from build123d import *

# Parameters (mm, degrees)
SALIENTE_EXTRUIR1_DEPTH = 18
SALIENTE_EXTRUIR6_START = -36
SALIENTE_EXTRUIR6_DEPTH = 66
CORTAR_EXTRUIR1_START   = 48
CORTAR_EXTRUIR1_DEPTH   = 46
CORTAR_EXTRUIR2_START   = 18
CROQUIS4_R              = 25
CORTAR_EXTRUIR2_DEPTH   = 340.524582953
CROQUIS5_W              = 115
CROQUIS5_H              = 90
SALIENTE_EXTRUIR7_DEPTH = 34.5
CORTAR_EXTRUIR3_START   = 72
CROQUIS7_R              = 20
CORTAR_EXTRUIR3_DEPTH   = 398.972479579


with BuildPart() as part:
    # Croquis1 → Saliente-Extruir1 (new, symmetric)
    with BuildSketch(Plane(origin=(0, 0, 0), x_dir=(1, 0, 0), z_dir=(0, 1, 0))):
        with BuildLine():
            Line((-194.323843522, -100.327234865), (201.676156478, -100.327234865))
            ThreePointArc((201.676156478, -100.327234865), (301.676156478, -0.327234865), (201.676156478, 99.672765135))
            Line((201.676156478, 99.672765135), (-194.323843522, 99.672765135))
            ThreePointArc((-194.323843522, 99.672765135), (-294.323843522, -0.327234865), (-194.323843522, -100.327234865))
        make_face()
    extrude(amount=SALIENTE_EXTRUIR1_DEPTH, both=True)

    # Croquis2 → Saliente-Extruir6 (add)
    with BuildSketch(Plane(origin=(0, 18, 0), x_dir=(1, 0, 0), z_dir=(0, 1, 0)).offset(SALIENTE_EXTRUIR6_START)):
        with BuildLine():
            Line((-194.323843522, -75.327234865), (201.676156478, -75.327234865))
            ThreePointArc((201.676156478, -75.327234865), (276.676156478, -0.327234865), (201.676156478, 74.672765135))
            Line((201.676156478, 74.672765135), (-194.323843522, 74.672765135))
            ThreePointArc((-194.323843522, 74.672765135), (-269.323843522, -0.327234865), (-194.323843522, -75.327234865))
        make_face()
    extrude(amount=SALIENTE_EXTRUIR6_DEPTH)

    # Croquis3 → Cortar-Extruir1 (cut)
    with BuildSketch(Plane(origin=(0, 0, 0), x_dir=(1, 0, 0), z_dir=(0, 1, 0)).offset(CORTAR_EXTRUIR1_START)):
        with BuildLine():
            Line((-194.323843522, -50.327234865), (201.676156478, -50.327234865))
            ThreePointArc((201.676156478, -50.327234865), (251.676156478, -0.327234865), (201.676156478, 49.672765135))
            Line((201.676156478, 49.672765135), (-194.323843522, 49.672765135))
            ThreePointArc((-194.323843522, 49.672765135), (-244.323843522, -0.327234865), (-194.323843522, -50.327234865))
        make_face()
    extrude(amount=-CORTAR_EXTRUIR1_DEPTH, mode=Mode.SUBTRACT)

    # Croquis4 → Cortar-Extruir2 (cut, through all)
    with BuildSketch(Plane(origin=(0, 0, 0), x_dir=(1, 0, 0), z_dir=(0, 1, 0)).offset(CORTAR_EXTRUIR2_START)):
        with Locations(Location((-194.323843522, -0.327234865, 0), (0, 0, 90))):
            Circle(CROQUIS4_R)
        with Locations(Location((201.676156478, -0.327234865, 0), (0, 0, 90))):
            Circle(CROQUIS4_R)
    extrude(amount=-CORTAR_EXTRUIR2_DEPTH, mode=Mode.SUBTRACT)

    # Croquis5 → Saliente-Extruir7 (add, symmetric)
    with BuildSketch(Plane.XY):
        with Locations((14.961556785, 27)):
            Rectangle(CROQUIS5_W, CROQUIS5_H)
    extrude(amount=SALIENTE_EXTRUIR7_DEPTH, both=True)

    # Croquis7 → Cortar-Extruir3 (cut, through all)
    with BuildSketch(Plane(origin=(0, 0, 0), x_dir=(1, 0, 0), z_dir=(0, 1, 0)).offset(CORTAR_EXTRUIR3_START)):
        with Locations(Location((12.367095305, 2.963956449, 0), (0, 0, 270))):
            Circle(CROQUIS7_R)
    extrude(amount=-CORTAR_EXTRUIR3_DEPTH, mode=Mode.SUBTRACT)


solid = part.part
For this review, take the finished solid that the model builds, in its own axes (mm). A direction names the side the tool comes from. Give positions to 0.01 mm unless a question says otherwise; leave off trailing zeros. Order: outer loops, then holes, each group sorted by start corner. A loop starts at its lowest first (then second) coordinate and runs counter-clockwise, first axis right, second up. Notation, with made-up numbers: (85, -33.75) - (141, -33.75) arc R28 cw to (141, 3.25) - close; hole circle Ø3 at (40.25, -31.75). An arc over 180 degrees is marked (long way). Answer as a JSON object with one key per item and string values. Group by question number.
Item 1: Machinability: for faces 1 (the flat face through (1, 33, 75.327)), 2 (the flat face through (1, 0, 100.327)), 3 (the flat face through (14, 37, -34.5)), which of the approach directions +Z, -Z, +X, -X, +Y, -Y give a long, thin tool a straight path to every point of the face, cutting with its end or side? Answer none if there is none.
Item 2: Wall thickness on line 1 along Z through (x, y) = (39, 30); line 2 along Z through (x, y) = (143.5, 19); line 3 along X through (y, z) = (19, -20.5): over which ranges is each line inside the solid? List them lowest first.
Item 3: Take a section at D-D on x = -203.5. Give the boundary of the cut face in (y, z).
Item 4: Take a section at B-B on x = -37. Give the boundary of the cut face in (y, z).
Item 5: Draft analysis for pull direction X (two halves, no side actions). For faces 4 (the cylindrical face through (276.658, 32.79, 1.976)), 5 (the flat face through (6, 33, -74.673)), 6 (the cylindrical face through (176.89, -7.86, 3.58)), state which applies: pulls with the +X half, pulls with the -X half, needs draft (parallel to the pull), parting line crosses it, or undercut.
Item 6: Clearance check with flat-ended pins moving along their axes: pin 1 Ø15 at (x, y) = (-50, 29.5) entering from +Z; pin 2 Ø3 at (y, z) = (28, 34.5) entering from +X; pin 3 Ø5 at (x, z) = (84, 64) entering from +Y. State where each tip first meets the part, or that it passes through.
Item 7: Take a section at C-C on y = -6. Give the boundary of the cut face in (x, z).
Item 8: Take a section at A-A on y = 37. Give the boundary of the cut face in (x, z).
Reported:
{
 "1": {"face 1": "+Z, +X, -X, +Y", "face 2": "+Z, +X, -X, +Y, -Y", "face 3": "+Y"},
 "2": {"line 1": "-74.67 to -49.67, -34.5 to 34.5, 50.33 to 75.33", "line 2": "-74.67 to -49.67, 50.33 to 75.33", "line 3": "-266.37 to -239.78, -42.54 to 2.75, 21.98 to 72.46, 247.13 to 273.73"},
 "3": {"outline": "(-18, -99.25) - (18, -99.25) - (18, -74.11) - (48, -74.11) - (48, -48.82) - (2, -48.82) - (2, -22.93) - (-18, -22.93) - close; (-18, 23.58) - (2, 23.58) - (2, 49.48) - (48, 49.48) - (48, 74.76) - (18, 74.76) - (18, 99.91) - (-18, 99.91) - close"},
 "4": {"outline": "(-18, -99.67) - (18, -99.67) - (18, -74.67) - (48, -74.67) - (48, -49.67) - (2, -49.67) - (2, -34.5) - (72, -34.5) - (72, 34.5) - (2, 34.5) - (2, 50.33) - (48, 50.33) - (48, 75.33) - (18, 75.33) - (18, 100.33) - (-18, 100.33) - close"},
 "5": {"face 4": "pulls with the +X half", "face 5": "needs draft", "face 6": "undercut"},
 "6": {"pin 1": "z = 75.33", "pin 2": "x = 269.19", "pin 3": "y = 48"},
 "7": {"outline": "(-194.32, -99.67) - (201.68, -99.67) arc R100 ccw to (201.68, 100.33) - (-194.32, 100.33) arc R100 ccw to start; hole circle Ø50 at (-194.32, 0.33); hole circle Ø40 at (12.37, -2.96); hole circle Ø50 at (201.68, 0.33)"},
 "8": {"outline": "(-194.32, -74.67) - (201.68, -74.67) arc R75 ccw to (201.68, 75.33) - (-194.32, 75.33) arc R75 ccw to start; (-42.54, -34.5) - (72.46, -34.5) - (72.46, 34.5) - (-42.54, 34.5) - close; hole (-194.32, -49.67) - (201.68, -49.67) arc R50 ccw to (201.68, 50.33) - (-194.32, 50.33) arc R50 ccw to start; hole circle Ø40 at (12.37, -2.96)"}
}
